The drawing under review shows one solid part. Ordinate dimensions are in mm from its lowest x, y, z. A direction names the side the tool comes from. Give positions to 0.01 mm unless a question says otherwise; leave off trailing zeros. Loops run counter-clockwise (first coordinate to the right, second up) from the corner with the lowest first, then second, coordinate; pieces in that order, holes last. Notation, with made-up numbers: (47.25, 62.25) - (105.25, 62.25) arc R31 ccw to (105.25, 94.25) - close; hole circle Ø2 at (9, 27.5). An arc over 180 degrees is marked (long way). Write each question's results on one line, items separated by ' | '.
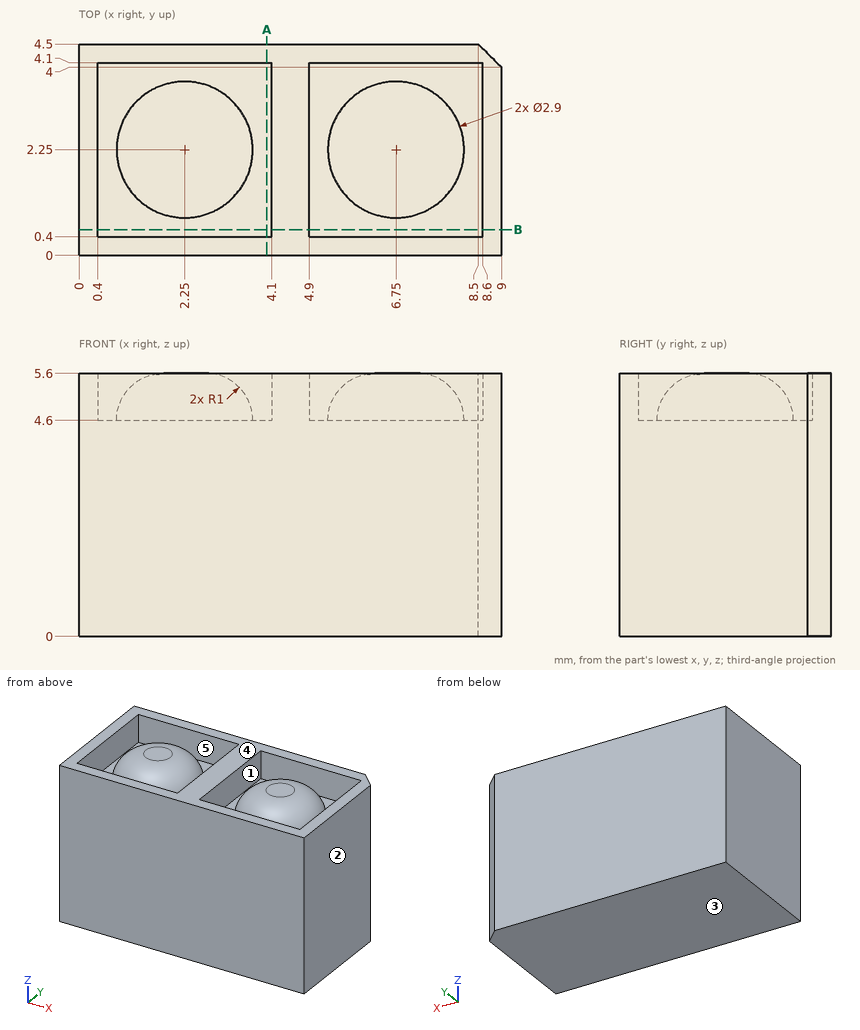
(1) Draft analysis for pull direction X (two halves, no side actions). For the marked faces 1, 2 and 3, state which applies: pulls with the +X half, pulls with the -X half, needs draft (parallel to the pull), parting line crosses it, or undercut.
Answers below:
face 1: undercut | face 2: pulls with the +X half | face 3: needs draft
(2) Take a section at B-B on y = 0.55. Give the boundary of the cut face in (x, z).
Answers below:
outline: (0, 0) - (9, 0) - (9, 5.6) - (8.6, 5.6) - (8.6, 4.6) - (4.9, 4.6) - (4.9, 5.6) - (4.1, 5.6) - (4.1, 4.6) - (0.4, 4.6) - (0.4, 5.6) - (0, 5.6) - close
(3) Take a section at A-A on x = 4. Give the boundary of the cut face in (y, z).
Answers below:
outline: (0, 0) - (4.5, 0) - (4.5, 5.6) - (4.1, 5.6) - (4.1, 4.6) - (0.4, 4.6) - (0.4, 5.6) - (0, 5.6) - close
(4) Wall thickness on line 1 along Z through (x, y) = (5, 1.35); line 2 along Z through (x, y) = (6, 1.45); line 3 along Y through (x, z) = (8.75, 4.2): over which ranges is each line inside the solid? List them lowest first. Write a range as from..to.
Answers below:
line 1: 0..4.6 | line 2: 0..5.36 | line 3: 0..4.25
(5) Insertion check: P1, Ø0.5, axis at x = 6.5, z = 5, coming from the -Y side. The pin has a flat end and moves straight along its axis. Give the tip position at first contact, or say it passes through.
Answers below:
P1: y = 0
(6) Tool access review of the marked faces 4 and 5: name each direction out of +Z, -Z, +X, -X, +Y, -Y from which nothing blocks a thin tool from reaching the whole face with its end or side.
Answers below:
face 4: +Z, +X, -X, +Y, -Y | face 5: +Z
